The listing builds one solid part. Answer for the finished solid, in the listing's coordinates (mm). A direction names the side the tool comes from. Give positions to 0.01 mm unless a question says otherwise; leave off trailing zeros. Write each loop counter-clockwise with the first axis right and the second up, starting at its lowest first coordinate (ties: lowest second). Pieces come first, ordered by that corner, then holes. Notation, with made-up numbers: M 38.5,-27.5 L 51.5,-27.5 A11 ccw 51.5,-23.5 Z; hole C 71.5,77 d6. An arc over 180 degrees is marked long. Answer as a JSON object with one key per item and string values.
```python
from build123d import *

# Parameters (mm, degrees)
SKETCH1_W           = 25.4
SKETCH1_H           = 25.4
BOSS_EXTRUDE1_DEPTH = 50.8
SKETCH2_R           = 1.8288
CUT_EXTRUDE1_DEPTH  = 12.7
SKETCH3_R           = 1.8288
CUT_EXTRUDE2_DEPTH  = 12.7


with BuildPart() as part:
    # Sketch1 → Boss-Extrude1 (new body)
    with BuildSketch(Plane(origin=(0, 0, 0), x_dir=(1, 0, 0), z_dir=(0, 1, 0))):
        Rectangle(SKETCH1_W, SKETCH1_H)
    extrude(amount=BOSS_EXTRUDE1_DEPTH)

    # Sketch2 → Cut-Extrude1 (cut)
    with BuildSketch(Plane(origin=(12.7, 0, 0), x_dir=(0, 0, -1), z_dir=(1, 0, 0))):
        with Locations((-6.35, 47.625)):
            Circle(SKETCH2_R)
        with Locations((6.35, 47.625)):
            Circle(SKETCH2_R)
        with Locations((6.35, 34.925)):
            Circle(SKETCH2_R)
        with Locations((-6.35, 34.925)):
            Circle(SKETCH2_R)
    extrude(amount=-CUT_EXTRUDE1_DEPTH, mode=Mode.SUBTRACT)

    # Sketch3 → Cut-Extrude2 (cut)
    with BuildSketch(Plane.XZ):
        with Locations((-6.35, 6.35)):
            Circle(SKETCH3_R)
        with Locations((6.35, 6.35)):
            Circle(SKETCH3_R)
        with Locations((6.35, -6.35)):
            Circle(SKETCH3_R)
        with Locations((-6.35, -6.35)):
            Circle(SKETCH3_R)
    extrude(amount=-CUT_EXTRUDE2_DEPTH, mode=Mode.SUBTRACT)


solid = part.part
```
1. The mould has two halves that part along X. Classify faces 1 (the cylindrical face through (-4.66, 6.26, 5.65)), 2 (the flat face through (0, 25, -12.7)), 3 (the flat face through (-6, 12.7, -6)), 4 (the flat face through (-12.7, 25, 0)): released by +X, released by -X, zero draft, split by the parting line, or undercut.
Verdict:
{"face 1": "undercut", "face 2": "zero draft", "face 3": "undercut", "face 4": "released by -X"}
2. A flat-ended cylindrical pin translates along its axis: pin 1 (1.1 mm diameter, centred on y = 48, z = -7, fed in from +X). Find the tip coordinate at first contact, or state that the pin passes through.
Verdict:
{"pin 1": "stops at x = 0"}
3. For faces 5 (the flat face through (6, 12.7, -6)), 6 (the flat face through (0, 0, 0)), 7 (the flat face through (0, 48, 6)), determine the directions among +Z, -Z, +X, -X, +Y, -Y from which every point of the face is accessible in a straight line to the end or side of a thin tool.
Verdict:
{"face 5": "-Y", "face 6": "+Z, -Z, +X, -X, -Y", "face 7": "+X"}
4. A cutting plane is placed at B-B, the plane y = 8.5. Give the vertices of the cut face in (x, z), plus the area to 3 significant figures.
Verdict:
{"outline": "M -12.7,-12.7 L 12.7,-12.7 L 12.7,12.7 L -12.7,12.7 Z; hole C -6.35,-6.35 d3.66; hole C -6.35,6.35 d3.66; hole C 6.35,-6.35 d3.66; hole C 6.35,6.35 d3.66", "area": "603 mm2"}
5. A cutting plane is placed at D-D, the plane z = 6.35. Give the vertices of the cut face in (x, y).
Verdict:
{"outline": "M -12.7,0 L -8.18,0 L -8.18,12.7 L -4.52,12.7 L -4.52,0 L 4.52,0 L 4.52,12.7 L 8.18,12.7 L 8.18,0 L 12.7,0 L 12.7,33.1 L 0,33.1 L 0,36.75 L 12.7,36.75 L 12.7,45.8 L 0,45.8 L 0,49.45 L 12.7,49.45 L 12.7,50.8 L -12.7,50.8 Z"}
6. A cutting plane is placed at A-A, the plane x = -6.35. Give the vertices of the cut face in (y, z).
Verdict:
{"outline": "M 0,-12.7 L 50.8,-12.7 L 50.8,12.7 L 0,12.7 L 0,8.18 L 12.7,8.18 L 12.7,4.52 L 0,4.52 L 0,-4.52 L 12.7,-4.52 L 12.7,-8.18 L 0,-8.18 Z"}
7. A cutting plane is placed at C-C, the plane x = 0.5. Give the vertices of the cut face in (y, z) (3 decimals), plus the area to 3 significant figures.
Verdict:
{"outline": "M 0,-12.7 L 50.8,-12.7 L 50.8,12.7 L 0,12.7 Z; hole C 34.925,-6.35 d3.658; hole C 34.925,6.35 d3.658; hole C 47.625,-6.35 d3.658; hole C 47.625,6.35 d3.658", "area": "1,250 mm2"}
8. Consider line 1 along Z through (x, y) = (6.35, 7.5); line 2 along Y through (x, z) = (4.25, 6.35); line 3 along Z through (x, y) = (5.5, 7). Determine where each line is inside the solid, lowest interval first.
Verdict:
{"line 1": "z = -12.7 to -8.18, -4.52 to 4.52, 8.18 to 12.7", "line 2": "y = 0 to 33.1, 36.75 to 45.8, 49.45 to 50.8", "line 3": "z = -12.7 to -7.97, -4.73 to 4.73, 7.97 to 12.7"}
